Design review of the part built by this model. Coordinates are the model's own, in mm. Face numbers are marked on the shaded views. A direction names the side the tool comes from. Round coordinates to 2 decimals unless told otherwise and drop trailing zeros. Loops run counter-clockwise (first coordinate to the right, second up) from the corner with the lowest first, then second, coordinate; pieces in that order, holes last. Notation, with made-up numbers: (79, 88.25) - (128, 88.25) arc R22 ccw to (128, 97.25) - close; hole circle Ø3 at (14.5, -35.5). An arc over 180 degrees is marked (long way). One line per question, with ' | ' between items. Start each with the question number.
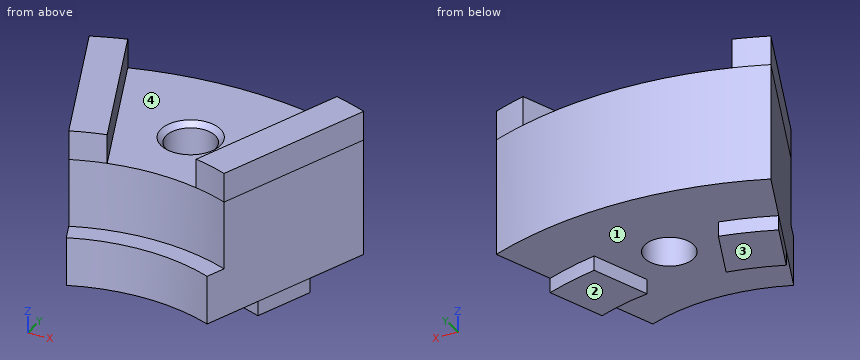
from build123d import *

# Parameters (mm, degrees)
BOSS_EXTRU_1_DEPTH          = 12
ENL_V_START                 = -7
ENL_V_MAT_EXTRU_1_DEPTH     = 7
BOSS_EXTRU_2_DEPTH          = 3
BOSS_EXTRU_3_DEPTH          = 1.5
TROU_TARAUD_M61_D           = 5
TROU_TARAUD_M61_CSINK_D     = 6.05
TROU_TARAUD_M61_CSINK_ANGLE = 90


with BuildPart() as part:
    # Esquisse2 → Boss.-Extru.1 (new body)
    with BuildSketch(Plane.XY):
        with BuildLine():
            Line((-7.146773921, 18.143142576), (-13.927046616, 35.355867583))
            ThreePointArc((-13.927046616, 35.355867583), (0, 38), (13.927046616, 35.355867583))
            Line((13.927046616, 35.355867583), (7.146773921, 18.143142576))
            ThreePointArc((7.146773921, 18.143142576), (0, 19.5), (-7.146773921, 18.143142576))
        make_face()
    extrude(amount=BOSS_EXTRU_1_DEPTH)

    # Esquisse4 → Enlèv. mat.-Extru.1 (cut)
    with BuildSketch(Plane.XY.offset(12).offset(ENL_V_START)):
        with BuildLine():
            Line((-7.879776375, 20.003977712), (-7.146773921, 18.143142576))
            ThreePointArc((-7.146773921, 18.143142576), (0, 19.5), (7.146773921, 18.143142576))
            Line((7.146773921, 18.143142576), (7.879776375, 20.003977712))
            ThreePointArc((7.879776375, 20.003977712), (0, 21.5), (-7.879776375, 20.003977712))
        make_face()
    extrude(amount=ENL_V_MAT_EXTRU_1_DEPTH, mode=Mode.SUBTRACT)

    # Esquisse5 → Boss.-Extru.2 (add)
    with BuildSketch(Plane.XY.offset(12)):
        with BuildLine():
            Line((-13.927046616, 35.355867583), (-7.879776375, 20.003977712))
            ThreePointArc((-7.879776375, 20.003977712), (-6.219766636, 20.580682763), (-4.518203594, 21.019891443))
            Line((-4.518203594, 21.019891443), (-10.611385095, 36.488333839))
            ThreePointArc((-10.611385095, 36.488333839), (-12.282274938, 35.960335404), (-13.927046616, 35.355867583))
        make_face()
        with BuildLine():
            Line((7.879776375, 20.003977712), (13.927046616, 35.355867583))
            ThreePointArc((13.927046616, 35.355867583), (12.282274938, 35.960335404), (10.611385095, 36.488333839))
            Line((10.611385095, 36.488333839), (4.518203594, 21.019891443))
            ThreePointArc((4.518203594, 21.019891443), (6.219766636, 20.580682763), (7.879776375, 20.003977712))
        make_face()
    extrude(amount=BOSS_EXTRU_2_DEPTH)

    # Esquisse6 → Boss.-Extru.3 (add)
    with BuildSketch(Plane(origin=(0, 0, 0), x_dir=(-1, 0, 0), z_dir=(0, 0, -1))):
        with BuildLine():
            Line((11.591313455, 29.42626351), (9.345781281, 23.725647984))
            ThreePointArc((9.345781281, 23.725647984), (6.716786511, 24.599487372), (4.008510327, 25.182967358))
            Line((4.008510327, 25.182967358), (6.297398832, 30.993649345))
            ThreePointArc((6.297398832, 30.993649345), (8.978623581, 30.325696206), (11.591313455, 29.42626351))
        make_face()
        with BuildLine():
            Line((-9.345781281, 23.725647984), (-11.591313455, 29.42626351))
            ThreePointArc((-11.591313455, 29.42626351), (-8.978623581, 30.325696206), (-6.297398832, 30.993649345))
            Line((-6.297398832, 30.993649345), (-4.008510327, 25.182967358))
            ThreePointArc((-4.008510327, 25.182967358), (-6.716786511, 24.599487372), (-9.345781281, 23.725647984))
        make_face()
    extrude(amount=BOSS_EXTRU_3_DEPTH)

    # Trou taraudé M61 (through all)
    with Locations(Plane.XY.offset(12)):
        with Locations((0, 28.5)):
            CounterSinkHole(TROU_TARAUD_M61_D / 2, TROU_TARAUD_M61_CSINK_D / 2, counter_sink_angle=TROU_TARAUD_M61_CSINK_ANGLE)


solid = part.part
1. Take a section at A-A, the plane x = 0. Give the boundary of the cut face in (y, z) (3 decimals).
2. Take a section at C-C, the plane z = 13.25. Give the boundary of the cut face in (x, y).
3. Take a section at D-D, the plane y = 28.5. Give the boundary of the cut face in (x, z) (3 decimals).
4. The part is to be moulded in two halves that separate along X. For the marked faces 1 and 2, say which applies: pulls with the +X half, pulls with the -X half, needs draft (parallel to the pull), parting line crosses it, or undercut.
5. Clearance check with flat-ended pins moving along their axes: P1, Ø1.7, axis at x = 3, y = 19.5, coming from the +Z side; P2, Ø1.5, axis at x = -7, z = 4.5, coming from the +Y side; P3, Ø6.5, axis at x = 0, y = 28.5, coming from the -Z side. State where each tip first meets the part, or that it passes through.
6. Machinability: for the marked faces 3 and 4, which of the approach directions +Z, -Z, +X, -X, +Y, -Y give a long, thin tool a straight path to every point of the face, cutting with its end or side? Answer none if there is none.
7. To check wall thickness, follow line 1 along Y through (x, z) = (0, 7); line 2 along Y through (x, z) = (0, 3.75); line 3 along Z through (x, y) = (5.5, 22). State the ranges of each line that lie inside material, in increasing order.
8. Take a section at B-B, the plane z = 4.25. Give the boundary of the cut face in (x, y), then the cut area to 3 significant figures.
Answer list:
1) outline: (19.5, 0) - (26, 0) - (26, 11.475) - (25.475, 12) - (21.5, 12) - (21.5, 5) - (19.5, 5) - close; (31, 0) - (38, 0) - (38, 12) - (31.525, 12) - (31, 11.475) - close
2) outline: (-13.93, 35.36) - (-7.88, 20) arc R21.5 cw to (-4.52, 21.02) - (-10.61, 36.49) arc R38 ccw to start; (4.52, 21.02) arc R21.5 cw to (7.88, 20) - (13.93, 35.36) arc R38 ccw to (10.61, 36.49) - close
3) outline: (-11.226, -1.5) - (-5.315, -1.5) - (-5.315, 0) - (-2.5, 0) - (-2.5, 11.475) - (-3.025, 12) - (-7.465, 12) - (-7.465, 15) - (-11.226, 15) - close; (2.5, 0) - (5.315, 0) - (5.315, -1.5) - (11.226, -1.5) - (11.226, 15) - (7.465, 15) - (7.465, 12) - (3.025, 12) - (2.5, 11.475) - close
4) face 1: undercut | face 2: needs draft
5) P1: stops at z = 5 | P2: stops at y = 37.48 | P3: stops at z = 0
6) face 3: -Z, +X, -X, +Y, -Y | face 4: +Z, +Y
7) line 1: y = 21.5 to 26, 31 to 38 | line 2: y = 19.5 to 26, 31 to 38 | line 3: z = 0 to 15
8) outline: (-13.93, 35.36) - (-7.15, 18.14) arc R19.5 cw to (7.15, 18.14) - (13.93, 35.36) arc R38 ccw to start; hole circle Ø5 at (0, 28.5) | area: 380 mm²
